```python
from build123d import *

# Parameters (mm, degrees)
SKETCH1_R           = 2.75
SKETCH1_W           = 130
SKETCH1_H           = 38
BOSS_EXTRUDE1_DEPTH = 10
SKETCH1_2_W         = 130
SKETCH1_2_H         = 38
BOSS_EXTRUDE2_DEPTH = 10
SKETCH14_W          = 15
SKETCH14_H          = 36
SKETCH14_W_2        = 104
SKETCH14_H_2        = 9
CUT_EXTRUDE2_DEPTH  = 77.811457479
FILLET2_R           = 4
SKETCH15_R          = 2.75
BOSS_EXTRUDE3_DEPTH = 40


with BuildPart() as part:
    # Sketch1 → Boss-Extrude1 (new body)
    with BuildSketch(Plane(origin=(0, 0, 0), x_dir=(1, 0, 0), z_dir=(0, 1, 0))):
        with BuildLine():
            Line((67, 30), (-67, 30))
            ThreePointArc((-67, 30), (-69.121320344, 29.121320344), (-70, 27))
            Line((-70, 27), (-70, -27))
            ThreePointArc((-70, -27), (-69.121320344, -29.121320344), (-67, -30))
            Line((-67, -30), (67, -30))
            ThreePointArc((67, -30), (69.121320344, -29.121320344), (70, -27))
            Line((70, -27), (70, 27))
            ThreePointArc((70, 27), (69.121320344, 29.121320344), (67, 30))
        make_face()
        with Locations(Location((-60, 24, 0), (0, 0, 270))):
            Circle(SKETCH1_R, mode=Mode.SUBTRACT)
        with Locations(Location((-60, -24, 0), (0, 0, 270))):
            Circle(SKETCH1_R, mode=Mode.SUBTRACT)
        with Locations(Location((60, -24, 0), (0, 0, 270))):
            Circle(SKETCH1_R, mode=Mode.SUBTRACT)
        with Locations(Location((60, 24, 0), (0, 0, 270))):
            Circle(SKETCH1_R, mode=Mode.SUBTRACT)
        Rectangle(SKETCH1_W, SKETCH1_H, mode=Mode.SUBTRACT)
    extrude(amount=BOSS_EXTRUDE1_DEPTH)

    # Sketch1<2> → Boss-Extrude2 (add)
    with BuildSketch(Plane(origin=(0, 0, 0), x_dir=(1, 0, 0), z_dir=(0, 1, 0))):
        Rectangle(SKETCH1_2_W, SKETCH1_2_H)
    extrude(amount=BOSS_EXTRUDE2_DEPTH)

    # Sketch14 → Cut-Extrude2 (cut, through all)
    with BuildSketch(Plane(origin=(0, 10, 0), x_dir=(1, 0, 0), z_dir=(0, 1, 0))):
        with Locations((-59.5, 0)):
            Rectangle(SKETCH14_W, SKETCH14_H)
        Rectangle(SKETCH14_W_2, SKETCH14_H)
        with Locations((0, 22.5)):
            Rectangle(SKETCH14_W_2, SKETCH14_H_2)
        with Locations((59.5, 0)):
            Rectangle(SKETCH14_W, SKETCH14_H)
        with Locations((0, -22.5)):
            Rectangle(SKETCH14_W_2, SKETCH14_H_2)
    extrude(amount=-CUT_EXTRUDE2_DEPTH, mode=Mode.SUBTRACT)

    # Fillet2
    fillet2_edges = [part.edges().sort_by_distance(p)[0] for p in [
        (-67, 5, 18),
        (-67, 5, -18),
        (-52, 5, -18),
        (-52, 5, -27),
        (52, 5, -27),
        (52, 5, -18),
        (67, 5, -18),
        (67, 5, 18),
        (52, 5, 18),
        (52, 5, 27),
        (-52, 5, 27),
        (-52, 5, 18),
    ]]
    fillet(fillet2_edges, radius=FILLET2_R)

    # Sketch15 → Boss-Extrude3 (add)
    with BuildSketch(Plane(origin=(0, 10, 0), x_dir=(1, 0, 0), z_dir=(0, 1, 0))):
        with BuildLine():
            Line((67, 30), (-67, 30))
            ThreePointArc((-67, 30), (-69.121320344, 29.121320344), (-70, 27))
            Line((-70, 27), (-70, -27))
            ThreePointArc((-70, -27), (-69.121320344, -29.121320344), (-67, -30))
            Line((-67, -30), (67, -30))
            ThreePointArc((67, -30), (69.121320344, -29.121320344), (70, -27))
            Line((70, -27), (70, 27))
            ThreePointArc((70, 27), (69.121320344, 29.121320344), (67, 30))
        make_face()
        with Locations(Location((-60, 24, 0), (0, 0, 270))):
            Circle(SKETCH15_R, mode=Mode.SUBTRACT)
        with Locations(Location((-60, -24, 0), (0, 0, 270))):
            Circle(SKETCH15_R, mode=Mode.SUBTRACT)
        with Locations(Location((60, -24, 0), (0, 0, 270))):
            Circle(SKETCH15_R, mode=Mode.SUBTRACT)
        with Locations(Location((60, 24, 0), (0, 0, 270))):
            Circle(SKETCH15_R, mode=Mode.SUBTRACT)
        with BuildLine():
            Line((56, -18), (63, -18))
            ThreePointArc((63, -18), (65.828427125, -16.828427125), (67, -14))
            Line((67, -14), (67, 14))
            ThreePointArc((67, 14), (65.828427125, 16.828427125), (63, 18))
            Line((63, 18), (56, 18))
            ThreePointArc((56, 18), (53.171572875, 19.171572875), (52, 22))
            Line((52, 22), (52, 23))
            ThreePointArc((52, 23), (50.828427125, 25.828427125), (48, 27))
            Line((48, 27), (-48, 27))
            ThreePointArc((-48, 27), (-50.828427125, 25.828427125), (-52, 23))
            Line((-52, 23), (-52, 22))
            ThreePointArc((-52, 22), (-53.171572875, 19.171572875), (-56, 18))
            Line((-56, 18), (-63, 18))
            ThreePointArc((-63, 18), (-65.828427125, 16.828427125), (-67, 14))
            Line((-67, 14), (-67, -14))
            ThreePointArc((-67, -14), (-65.828427125, -16.828427125), (-63, -18))
            Line((-63, -18), (-56, -18))
            ThreePointArc((-56, -18), (-53.171572875, -19.171572875), (-52, -22))
            Line((-52, -22), (-52, -23))
            ThreePointArc((-52, -23), (-50.828427125, -25.828427125), (-48, -27))
            Line((-48, -27), (48, -27))
            ThreePointArc((48, -27), (50.828427125, -25.828427125), (52, -23))
            Line((52, -23), (52, -22))
            ThreePointArc((52, -22), (53.171572875, -19.171572875), (56, -18))
        make_face(mode=Mode.SUBTRACT)
    extrude(amount=BOSS_EXTRUDE3_DEPTH)


solid = part.part
```
Geometry: final body of the model. Coordinates: model frame, mm. A direction names the side the tool comes from. Round coordinates to 2 decimals unless told otherwise and drop trailing zeros. Loops run counter-clockwise (first coordinate to the right, second up) from the corner with the lowest first, then second, coordinate; pieces in that order, holes last. Notation, with made-up numbers: (-22.75, 18) -> (27.25, 18) arc R19 cw to (27.25, 23) -> close; hole circle Ø7 at (-2, -16.5). An arc over 180 degrees is marked (long way). Write each question's results on one line, items separated by ' | '.
Item 1: Pull-direction query (Z, two-part tool) for faces 1 (the face through (-69.14, 24.65, 29.1)), 2 (the face through (-67, 25, 0)), 3 (the face through (60, 25, -18)), 4 (the face through (0, 0, 29)); classes: pulls with the +Z half, pulls with the -Z half, needs draft (parallel to the pull), parting line crosses it, or undercut.
Answers below:
face 1: pulls with the +Z half | face 2: undercut | face 3: undercut | face 4: needs draft
Item 2: Pin query (flat end, axial travel): pin 1 Ø6.5 at (x, z) = (-60, 24) entering from +Y; pin 2 Ø5 at (x, z) = (-60, -24) entering from -Y. Return the tip coordinate at first contact, or that it passes through.
Answers below:
pin 1: stops at y = 50 | pin 2: passes through
Item 3: Set-up query: faces 5 (the face through (-70, 25, 0)), 6 (the face through (59, 25, 18)). Return all of +Z, -Z, +X, -X, +Y, -Y with unobstructed straight access to the full face (end or side cutting, diameter ignored); none if empty.
Answers below:
face 5: +Z, -Z, -X, +Y, -Y | face 6: +Y, -Y
Item 4: Cut plane A-A on z = 6. Return the cut outline in (x, y).
Answers below:
outline: (-70, 0) -> (-67, 0) -> (-67, 50) -> (-70, 50) -> close; (67, 0) -> (70, 0) -> (70, 50) -> (67, 50) -> close
Item 5: Cut plane C-C on x = -41. Return the cut outline in (y, z).
Answers below:
outline: (0, -30) -> (50, -30) -> (50, -27) -> (0, -27) -> close; (0, 27) -> (50, 27) -> (50, 30) -> (0, 30) -> close
Item 6: Line query: probe 1 along Z at (x, y) = (39, 17.5); probe 2 along X at (y, z) = (6.5, -1); probe 3 along X at (y, z) = (21.5, 26). Output: solid intervals per line, ascending. Write a range as [from, to].
Answers below:
probe 1: z = [-30, -27], [27, 30] | probe 2: x = [-70, -67], [67, 70] | probe 3: x = [-70, -61.89], [-58.11, -50.65], [50.65, 58.11], [61.89, 70]
Item 7: Cut plane D-D on z = -25. Return the cut outline in (x, y).
Answers below:
outline: (-70, 0) -> (-62.56, 0) -> (-62.56, 50) -> (-70, 50) -> close; (-57.44, 0) -> (-51.46, 0) -> (-51.46, 50) -> (-57.44, 50) -> close; (51.46, 0) -> (57.44, 0) -> (57.44, 50) -> (51.46, 50) -> close; (62.56, 0) -> (70, 0) -> (70, 50) -> (62.56, 50) -> close
Item 8: Cut plane B-B on x = 60. Return the cut outline in (y, z), and give its area (3 significant figures).
Answers below:
outline: (0, -30) -> (50, -30) -> (50, -26.75) -> (0, -26.75) -> close; (0, -21.25) -> (50, -21.25) -> (50, -18) -> (0, -18) -> close; (0, 18) -> (50, 18) -> (50, 21.25) -> (0, 21.25) -> close; (0, 26.75) -> (50, 26.75) -> (50, 30) -> (0, 30) -> close | area: 650 mm²
